from build123d import *

# Parameters (mm, degrees)
EXTRUDE_1_DEPTH     = 35
SKETCH_2_W          = 54.5
SKETCH_2_H          = 30.5
SKETCH_2_R          = 1.75
EXTRUDE_2_DEPTH     = 3
CUT_EXTRUDE_2_DEPTH = 63.069014009


with BuildPart() as part:
    # Эскиз1 → Бобышка-Вытянуть1 (new body)
    with BuildSketch(Plane.XY):
        with BuildLine():
            Line((-32, 0), (-35, 0))
            Line((-35, 0), (-35, -25))
            Line((-35, -25), (0, -25))
            Line((0, -25), (0, 0))
            Line((0, 0), (-3, 0))
            ThreePointArc((-3, 0), (-17.5, -14.5), (-32, 0))
        make_face()
    extrude(amount=EXTRUDE_1_DEPTH)

    # Эскиз2 → Бобышка-Вытянуть2 (add)
    with BuildSketch(Plane.XY.offset(35)):
        with Locations((-17.5, -9.75)):
            Rectangle(SKETCH_2_W, SKETCH_2_H)
        with Locations((6.9, 0)):
            Circle(SKETCH_2_R, mode=Mode.SUBTRACT)
        with Locations(Location((-41.9, 0, 0), (0, 0, 180))):
            Circle(SKETCH_2_R, mode=Mode.SUBTRACT)
    extrude(amount=EXTRUDE_2_DEPTH)

    # Эскиз3 → Вырез-Вытянуть2 (cut, through all)
    with BuildSketch(Plane(origin=(0, 0, 35), x_dir=(-1, 0, 0), z_dir=(0, 0, -1))):
        with BuildLine():
            Line((3, 0), (0, 5.5))
            Line((0, 5.5), (35, 5.5))
            Line((35, 5.5), (32, 0))
            ThreePointArc((32, 0), (17.5, -14.5), (3, 0))
        make_face()
    extrude(amount=-CUT_EXTRUDE_2_DEPTH, mode=Mode.SUBTRACT)


solid = part.part
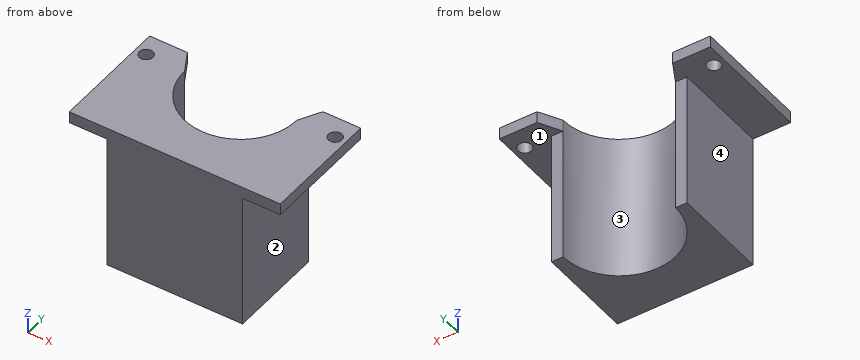
For this review, take the finished solid that the model builds, in its own axes (mm). Face numbers are marked on the shaded views. Round coordinates to 2 decimals unless told otherwise and drop trailing zeros. Loops run counter-clockwise (first coordinate to the right, second up) from the corner with the lowest first, then second, coordinate; pieces in that order, holes last. Notation, with made-up numbers: (55.25, -9.5) - (81.25, -9.5) arc R13 cw to (81.25, -2.5) - close; hole circle Ø11 at (-20.75, 2.25). An arc over 180 degrees is marked (long way). Use one line per item in the form item = value.
Item 1: Consider section D-D on x = -28. Write out the cut boundary in (y, z), then the cut area to 3 significant figures.
Answers:
outline = (-25, 0) - (-10, 0) - (-10, 38) - (-25, 38) - close
area = 570 mm^2
Item 2: Consider section A-A on x = 6.9. Write out the cut boundary in (y, z).
Answers:
outline = (-25, 35) - (-1.75, 35) - (-1.75, 38) - (-25, 38) - close; (1.75, 35) - (5.5, 35) - (5.5, 38) - (1.75, 38) - close
Item 3: Consider section C-C on z = 22. Write out the cut boundary in (x, y), then the cut area to 3 significant figures.
Answers:
outline = (-35, -25) - (0, -25) - (0, 0) - (-3, 0) arc R14.5 cw to (-32, 0) - (-35, 0) - close
area = 545 mm^2
Item 4: Clearance check with flat-ended pins moving along their axes: P1, Ø1.5, axis at x = -1.5, z = 14.5, coming from the +Y side; P2, Ø1.5, axis at x = -10.5, z = 27, coming from the +Y side; P3, Ø4, axis at x = 4, y = -16, coming from the -Z side. State where each tip first meets the part, or that it passes through.
Answers:
P1 = 0
P2 = -12.26
P3 = 35
Item 5: Mouldability with a two-part tool opening along X and no side actions: class the marked faces 1, 2, 3 and 4 as +X half, -X half, draft (parallel to the pull), parting line (faces both ways), or undercut.
Answers:
face_1 = draft
face_2 = +X half
face_3 = undercut
face_4 = -X half
Item 6: For line 1 (Y direction, x = 6.9, z = 35.95); line 2 (X direction, y = -24, z = 32); line 3 (Y direction, x = -0.5, z = 22.5), list the stretches that pass through material, from the lowest coordinate up.
Answers:
line_1 = -25 to -1.75, 1.75 to 5.5
line_2 = -35 to 0
line_3 = -25 to 0
Item 7: Consider section B-B on y = -7.5. Write out the cut boundary in (x, z), then the cut area to 3 significant figures.
Answers:
outline = (-44.75, 35) - (-35, 35) - (-35, 0) - (-29.91, 0) - (-29.91, 38) - (-44.75, 38) - close; (-5.09, 0) - (0, 0) - (0, 35) - (9.75, 35) - (9.75, 38) - (-5.09, 38) - close
area = 445 mm^2
